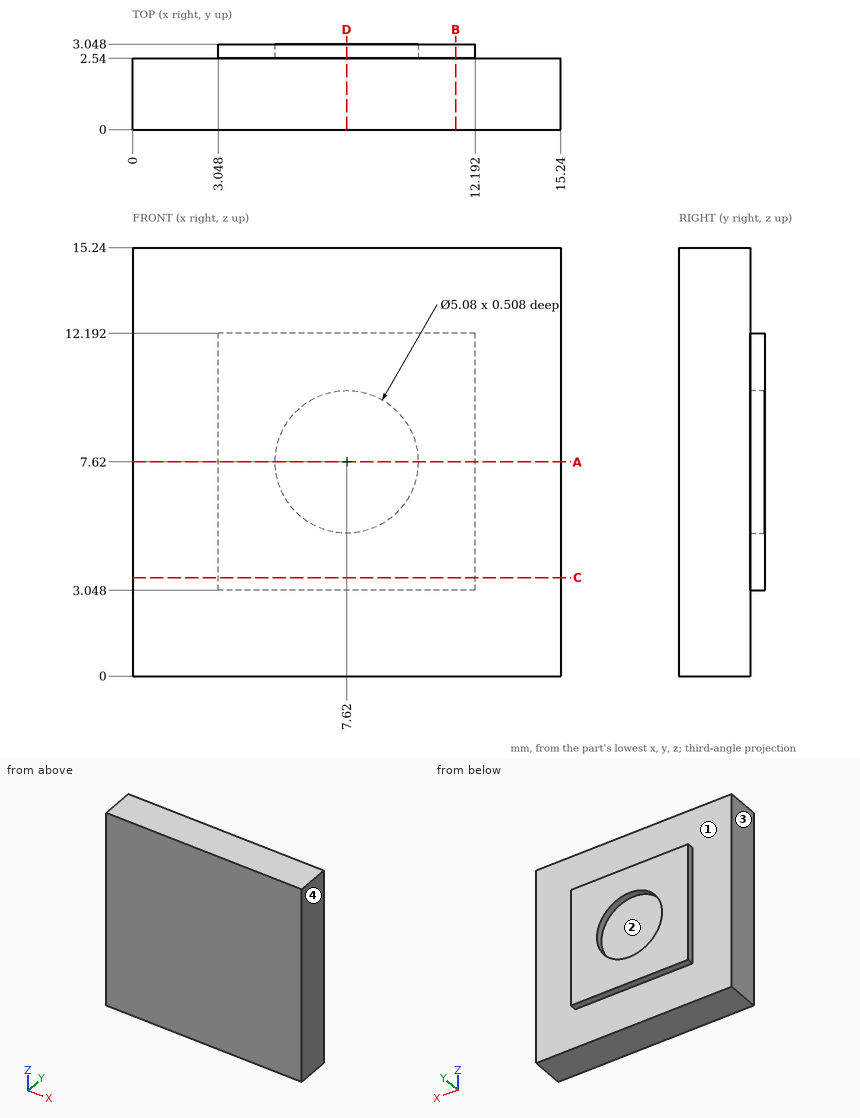
Job drawing, mm, ordinate dimensions from the low corner. One solid piece. Coordinates: 2 decimals unless noted, no trailing zeros. Order: outer loops, then holes, each group sorted by start corner. A loop starts at its lowest first (then second) coordinate and runs counter-clockwise, first axis right, second up. Notation, with made-up numbers: (85, 85) - (138, 85) arc R20 cw to (138, 114) - close; hole circle Ø1 at (-30, 20.5). An arc over 180 degrees is marked (long way). Return JSON: item names as keys, results as strings. Group by question number.
1) Saw through at D-D, the plane x = 7.62. Write the cut outline in (y, z).
2) Probe line 1 (Z direction, x = 7.62, y = 2.9); line 2 (Y direction, x = 13.75, z = 11.75). List the from-to ranges inside material, lowest first. Write a range as from..to.
3) Mould opens along X. For the marked faces 1, 2, 3 and 4 say: released by +X, released by -X, zero draft, split by the parting line, or undercut.
4) Saw through at B-B, the plane x = 11.5. Write the cut outline in (y, z), plus the area to 3 significant figures.
5) Saw through at C-C, the plane z = 3.5. Write the cut outline in (x, y).
6) Saw through at A-A, the plane z = 7.62. Write the cut outline in (x, y), plus the area to 3 significant figures.
7) Flat gauge pins, fed straight in: P1, Ø5, axis at x = 2.5, z = 3, coming from the -Y side; P2, Ø0.6, axis at y = 3, z = 10, coming from the -X side; P3, Ø1.5, axis at x = 8, z = 6.5, coming from the +Y side. Where does each tip first touch, or does it go through?
Values found:
{
 "1": {"outline": "(0, 0) - (2.54, 0) - (2.54, 3.05) - (3.05, 3.05) - (3.05, 5.08) - (2.54, 5.08) - (2.54, 10.16) - (3.05, 10.16) - (3.05, 12.19) - (2.54, 12.19) - (2.54, 15.24) - (0, 15.24) - close"},
 "2": {"line 1": "z = 3.05..5.08, 10.16..12.19", "line 2": "y = 0..2.54"},
 "3": {"face 1": "zero draft", "face 2": "undercut", "face 3": "released by -X", "face 4": "released by +X"},
 "4": {"outline": "(0, 0) - (2.54, 0) - (2.54, 3.05) - (3.05, 3.05) - (3.05, 12.19) - (2.54, 12.19) - (2.54, 15.24) - (0, 15.24) - close", "area": "43.4 mm²"},
 "5": {"outline": "(0, 0) - (15.24, 0) - (15.24, 2.54) - (12.19, 2.54) - (12.19, 3.05) - (3.05, 3.05) - (3.05, 2.54) - (0, 2.54) - close"},
 "6": {"outline": "(0, 0) - (15.24, 0) - (15.24, 2.54) - (12.19, 2.54) - (12.19, 3.05) - (10.16, 3.05) - (10.16, 2.54) - (5.08, 2.54) - (5.08, 3.05) - (3.05, 3.05) - (3.05, 2.54) - (0, 2.54) - close", "area": "40.8 mm²"},
 "7": {"P1": "stops at y = 0", "P2": "stops at x = 3.05", "P3": "stops at y = 2.54"}
}
